Input: part model. Units: mm. Frame: model coordinates. Give positions to 0.01 mm unless a question says otherwise; leave off trailing zeros. Order: outer loops, then holes, each group sorted by start corner. A loop starts at its lowest first (then second) coordinate and runs counter-clockwise, first axis right, second up. Notation, with made-up numbers: (63.5, 75) - (110.5, 75) arc R12 cw to (110.5, 96) - close; hole circle Ø6 at (57, -15.75). An arc over 180 degrees is marked (long way). Use a Markdown table: item, result.
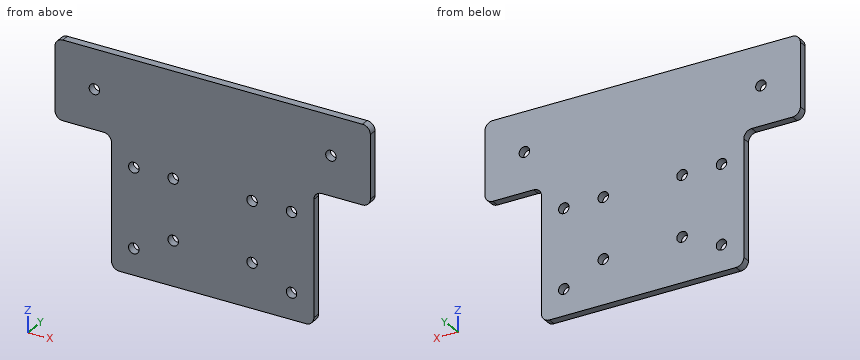
from build123d import *

# Parameters (mm, degrees)
SZKIC1_W                    = 77
SZKIC1_H                    = 80
DODANIE_WYCI_GNI_CIE1_DEPTH = 3
WYTNIJ_WYCI_GNI_CIE1_REACH  = 57.599
SZKIC2_R                    = 2.5
SZKIC2_R_2                  = 2
ZAOKR_GLENIE1_R             = 3
ZAOKR_GLENIE2_R             = 3
WYTNIJ_WYCI_GNI_CIE3_REACH  = 57.599
SZKIC3_R                    = 2
SZKIC5_W                    = 120
SZKIC5_H                    = 30
DODANIE_WYCI_GNI_CIE2_DEPTH = 3
ZAOKR_GLENIE4_R             = 3
WYTNIJ_WYCI_GNI_CIE4_REACH  = 74.173
SZKIC6_R                    = 2


with BuildPart() as part:
    # Szkic1 → Dodanie-wyciągnięcie1 (new body)
    with BuildSketch(Plane(origin=(0, 0, 0), x_dir=(1, 0, 0), z_dir=(0, 1, 0))):
        Rectangle(SZKIC1_W, SZKIC1_H)
    extrude(amount=DODANIE_WYCI_GNI_CIE1_DEPTH)

    # Szkic2 → Wytnij-wyciągnięcie1 (cut, up to next)
    with BuildSketch(Plane(origin=(0, 3, 0), x_dir=(1, 0, 0), z_dir=(0, 1, 0)), mode=Mode.PRIVATE) as wytnij_wyci_gni_cie1_sk1:
        with Locations(Location((-23.5, -25, 0), (0, 0, 270))):
            Circle(SZKIC2_R)
    wytnij_wyci_gni_cie1_tool1 = extrude(wytnij_wyci_gni_cie1_sk1.sketch, amount=-WYTNIJ_WYCI_GNI_CIE1_REACH, mode=Mode.PRIVATE) & part.part
    # Szkic2 → Wytnij-wyciągnięcie1 (cut, up to next)
    with BuildSketch(Plane(origin=(0, 3, 0), x_dir=(1, 0, 0), z_dir=(0, 1, 0)), mode=Mode.PRIVATE) as wytnij_wyci_gni_cie1_sk2:
        with Locations(Location((23.5, -25, 0), (0, 0, 270))):
            Circle(SZKIC2_R)
    wytnij_wyci_gni_cie1_tool2 = extrude(wytnij_wyci_gni_cie1_sk2.sketch, amount=-WYTNIJ_WYCI_GNI_CIE1_REACH, mode=Mode.PRIVATE) & part.part
    # Szkic2 → Wytnij-wyciągnięcie1 (cut, up to next)
    with BuildSketch(Plane(origin=(0, 3, 0), x_dir=(1, 0, 0), z_dir=(0, 1, 0)), mode=Mode.PRIVATE) as wytnij_wyci_gni_cie1_sk3:
        with Locations(Location((-30, 30, 0), (0, 0, 270))):
            Circle(SZKIC2_R_2)
    wytnij_wyci_gni_cie1_tool3 = extrude(wytnij_wyci_gni_cie1_sk3.sketch, amount=-WYTNIJ_WYCI_GNI_CIE1_REACH, mode=Mode.PRIVATE) & part.part
    # Szkic2 → Wytnij-wyciągnięcie1 (cut, up to next)
    with BuildSketch(Plane(origin=(0, 3, 0), x_dir=(1, 0, 0), z_dir=(0, 1, 0)), mode=Mode.PRIVATE) as wytnij_wyci_gni_cie1_sk4:
        with Locations(Location((-30, 0, 0), (0, 0, 270))):
            Circle(SZKIC2_R_2)
    wytnij_wyci_gni_cie1_tool4 = extrude(wytnij_wyci_gni_cie1_sk4.sketch, amount=-WYTNIJ_WYCI_GNI_CIE1_REACH, mode=Mode.PRIVATE) & part.part
    # Szkic2 → Wytnij-wyciągnięcie1 (cut, up to next)
    with BuildSketch(Plane(origin=(0, 3, 0), x_dir=(1, 0, 0), z_dir=(0, 1, 0)), mode=Mode.PRIVATE) as wytnij_wyci_gni_cie1_sk5:
        with Locations(Location((30, 0, 0), (0, 0, 270))):
            Circle(SZKIC2_R_2)
    wytnij_wyci_gni_cie1_tool5 = extrude(wytnij_wyci_gni_cie1_sk5.sketch, amount=-WYTNIJ_WYCI_GNI_CIE1_REACH, mode=Mode.PRIVATE) & part.part
    # Szkic2 → Wytnij-wyciągnięcie1 (cut, up to next)
    with BuildSketch(Plane(origin=(0, 3, 0), x_dir=(1, 0, 0), z_dir=(0, 1, 0)), mode=Mode.PRIVATE) as wytnij_wyci_gni_cie1_sk6:
        with Locations(Location((30, 30, 0), (0, 0, 270))):
            Circle(SZKIC2_R_2)
    wytnij_wyci_gni_cie1_tool6 = extrude(wytnij_wyci_gni_cie1_sk6.sketch, amount=-WYTNIJ_WYCI_GNI_CIE1_REACH, mode=Mode.PRIVATE) & part.part
    add(wytnij_wyci_gni_cie1_tool1.solids().sort_by_distance((-23.5, 3, 25))[0], mode=Mode.SUBTRACT)
    add(wytnij_wyci_gni_cie1_tool2.solids().sort_by_distance((23.5, 3, 25))[0], mode=Mode.SUBTRACT)
    add(wytnij_wyci_gni_cie1_tool3.solids().sort_by_distance((-30, 3, -30))[0], mode=Mode.SUBTRACT)
    add(wytnij_wyci_gni_cie1_tool4.solids().sort_by_distance((-30, 3, 0))[0], mode=Mode.SUBTRACT)
    add(wytnij_wyci_gni_cie1_tool5.solids().sort_by_distance((30, 3, 0))[0], mode=Mode.SUBTRACT)
    add(wytnij_wyci_gni_cie1_tool6.solids().sort_by_distance((30, 3, -30))[0], mode=Mode.SUBTRACT)

    # Zaokrąglenie1
    zaokr_glenie1_edges = [part.edges().sort_by_distance(p)[0] for p in [
        (-38.5, 1.5, -40),
    ]]
    fillet(zaokr_glenie1_edges, radius=ZAOKR_GLENIE1_R)

    # Zaokrąglenie2
    zaokr_glenie2_edges = [part.edges().sort_by_distance(p)[0] for p in [
        (38.5, 1.5, 40),
        (-38.5, 1.5, 40),
        (38.5, 1.5, -40),
    ]]
    fillet(zaokr_glenie2_edges, radius=ZAOKR_GLENIE2_R)

    # Szkic3 → Wytnij-wyciągnięcie3 (cut, up to next)
    with BuildSketch(Plane(origin=(0, 0, 0), x_dir=(1, 0, 0), z_dir=(0, 1, 0)), mode=Mode.PRIVATE) as wytnij_wyci_gni_cie3_sk1:
        with Locations(Location((-15, 23, 0), (0, 0, 90))):
            Circle(SZKIC3_R)
    wytnij_wyci_gni_cie3_tool1 = extrude(wytnij_wyci_gni_cie3_sk1.sketch, amount=WYTNIJ_WYCI_GNI_CIE3_REACH, mode=Mode.PRIVATE) & part.part
    # Szkic3 → Wytnij-wyciągnięcie3 (cut, up to next)
    with BuildSketch(Plane(origin=(0, 0, 0), x_dir=(1, 0, 0), z_dir=(0, 1, 0)), mode=Mode.PRIVATE) as wytnij_wyci_gni_cie3_sk2:
        with Locations(Location((15, 23, 0), (0, 0, 90))):
            Circle(SZKIC3_R)
    wytnij_wyci_gni_cie3_tool2 = extrude(wytnij_wyci_gni_cie3_sk2.sketch, amount=WYTNIJ_WYCI_GNI_CIE3_REACH, mode=Mode.PRIVATE) & part.part
    # Szkic3 → Wytnij-wyciągnięcie3 (cut, up to next)
    with BuildSketch(Plane(origin=(0, 0, 0), x_dir=(1, 0, 0), z_dir=(0, 1, 0)), mode=Mode.PRIVATE) as wytnij_wyci_gni_cie3_sk3:
        with Locations(Location((-15, 0, 0), (0, 0, 90))):
            Circle(SZKIC3_R)
    wytnij_wyci_gni_cie3_tool3 = extrude(wytnij_wyci_gni_cie3_sk3.sketch, amount=WYTNIJ_WYCI_GNI_CIE3_REACH, mode=Mode.PRIVATE) & part.part
    # Szkic3 → Wytnij-wyciągnięcie3 (cut, up to next)
    with BuildSketch(Plane(origin=(0, 0, 0), x_dir=(1, 0, 0), z_dir=(0, 1, 0)), mode=Mode.PRIVATE) as wytnij_wyci_gni_cie3_sk4:
        with Locations(Location((15, 0, 0), (0, 0, 90))):
            Circle(SZKIC3_R)
    wytnij_wyci_gni_cie3_tool4 = extrude(wytnij_wyci_gni_cie3_sk4.sketch, amount=WYTNIJ_WYCI_GNI_CIE3_REACH, mode=Mode.PRIVATE) & part.part
    add(wytnij_wyci_gni_cie3_tool1.solids().sort_by_distance((-15, 0, -23))[0], mode=Mode.SUBTRACT)
    add(wytnij_wyci_gni_cie3_tool2.solids().sort_by_distance((15, 0, -23))[0], mode=Mode.SUBTRACT)
    add(wytnij_wyci_gni_cie3_tool3.solids().sort_by_distance((-15, 0, 0))[0], mode=Mode.SUBTRACT)
    add(wytnij_wyci_gni_cie3_tool4.solids().sort_by_distance((15, 0, 0))[0], mode=Mode.SUBTRACT)

    # Szkic5 → Dodanie-wyciągnięcie2 (add)
    with BuildSketch(Plane(origin=(0, 3, 0), x_dir=(1, 0, 0), z_dir=(0, 1, 0))):
        with Locations((0, -25)):
            Rectangle(SZKIC5_W, SZKIC5_H)
    extrude(amount=-DODANIE_WYCI_GNI_CIE2_DEPTH)

    # Zaokrąglenie4
    zaokr_glenie4_edges = [part.edges().sort_by_distance(p)[0] for p in [
        (-60, 1.5, 10),
        (60, 1.5, 40),
        (-60, 1.5, 40),
        (38.5, 1.5, 10),
        (-38.5, 1.5, 10),
        (60, 1.5, 10),
    ]]
    fillet(zaokr_glenie4_edges, radius=ZAOKR_GLENIE4_R)

    # Szkic6 → Wytnij-wyciągnięcie4 (cut, up to next)
    with BuildSketch(Plane(origin=(0, 3, 0), x_dir=(1, 0, 0), z_dir=(0, 1, 0)), mode=Mode.PRIVATE) as wytnij_wyci_gni_cie4_sk1:
        with Locations(Location((-45, -25, 0), (0, 0, 270))):
            Circle(SZKIC6_R)
    wytnij_wyci_gni_cie4_tool1 = extrude(wytnij_wyci_gni_cie4_sk1.sketch, amount=-WYTNIJ_WYCI_GNI_CIE4_REACH, mode=Mode.PRIVATE) & part.part
    # Szkic6 → Wytnij-wyciągnięcie4 (cut, up to next)
    with BuildSketch(Plane(origin=(0, 3, 0), x_dir=(1, 0, 0), z_dir=(0, 1, 0)), mode=Mode.PRIVATE) as wytnij_wyci_gni_cie4_sk2:
        with Locations(Location((45, -25, 0), (0, 0, 270))):
            Circle(SZKIC6_R)
    wytnij_wyci_gni_cie4_tool2 = extrude(wytnij_wyci_gni_cie4_sk2.sketch, amount=-WYTNIJ_WYCI_GNI_CIE4_REACH, mode=Mode.PRIVATE) & part.part
    add(wytnij_wyci_gni_cie4_tool1.solids().sort_by_distance((-45, 3, 25))[0], mode=Mode.SUBTRACT)
    add(wytnij_wyci_gni_cie4_tool2.solids().sort_by_distance((45, 3, 25))[0], mode=Mode.SUBTRACT)


solid = part.part
1. Section query B-B (x = -30). Return loops of the section in (y, z), then the cut area to 3 significant figures.
Response:
| item | result |
|---|---|
| outline | (0, -40) - (3, -40) - (3, -32) - (0, -32) - close; (0, -28) - (3, -28) - (3, -2) - (0, -2) - close; (0, 2) - (3, 2) - (3, 40) - (0, 40) - close |
| area | 216 mm^2 |
2. Material intervals for line 1 along X through (y, z) = (1.9, 25); line 2 along X through (y, z) = (1.85, -30); line 3 along X through (y, z) = (2.3, 0), sorted ascending.
Response:
| item | result |
|---|---|
| line 1 | x = -60 to -47, -43 to 43, 47 to 60 |
| line 2 | x = -38.5 to -32, -28 to 28, 32 to 38.5 |
| line 3 | x = -38.5 to -32, -28 to -17, -13 to 13, 17 to 28, 32 to 38.5 |
3. Section query A-A (z = 25). Return loops of the section in (x, y).
Response:
| item | result |
|---|---|
| outline | (-60, 0) - (-47, 0) - (-47, 3) - (-60, 3) - close; (-43, 0) - (43, 0) - (43, 3) - (-43, 3) - close; (47, 0) - (60, 0) - (60, 3) - (47, 3) - close |
4. Section query D-D (z = 0). Return loops of the section in (x, y).
Response:
| item | result |
|---|---|
| outline | (-38.5, 0) - (-32, 0) - (-32, 3) - (-38.5, 3) - close; (-28, 0) - (-17, 0) - (-17, 3) - (-28, 3) - close; (-13, 0) - (13, 0) - (13, 3) - (-13, 3) - close; (17, 0) - (28, 0) - (28, 3) - (17, 3) - close; (32, 0) - (38.5, 0) - (38.5, 3) - (32, 3) - close |
5. Pin query (flat end, axial travel): pin 1 (3 mm diameter, centred on x = -30, z = 0, fed in from -Y); pin 2 (1.5 mm diameter, centred on y = 1.5, z = -21.5, fed in from +X); pin 3 (6.5 mm diameter, centred on x = -45, z = 25, fed in from -Y); pin 4 (1 mm diameter, centred on x = -37, y = 1, fed in from -Z). Return the tip coordinate at first contact, or that it passes through.
Response:
| item | result |
|---|---|
| pin 1 | passes through |
| pin 2 | stops at x = 38.5 |
| pin 3 | stops at y = 0 |
| pin 4 | stops at z = -39.83 |
6. Section query C-C (y = 0.5). State how many separate pieces and enclosed holes the cut face has, then the cut area to 3 significant figures.
Response:
| item | result |
|---|---|
| separate pieces | 1 |
| enclosed holes | 10 |
| area | 7,320 mm^2 |
